from build123d import *

# Parameters (mm, degrees)
F0_W     = 41
F0_H     = 41
F1_DEPTH = 47
F2_R     = 1.25
F3_DEPTH = 25
F4_R     = 11
F5_DEPTH = 2
F6_R     = 2.25
F7_DEPTH = 21
F8_R     = 8
F9_DEPTH = 7


with BuildPart() as f1:
    # F0 (on Top) → F1 (new body)
    with BuildSketch(Plane.XY):
        with Locations((20.5, 20.5)):
            Rectangle(F0_W, F0_H)
    extrude(amount=F1_DEPTH)

    # F2 (on face) → F3 (cut)
    with BuildSketch(Plane.XY.offset(47)):
        with Locations((5, 5)):
            Circle(F2_R)
        with Locations((36, 5)):
            Circle(F2_R)
        with Locations((36, 36)):
            Circle(F2_R)
        with Locations((5, 36)):
            Circle(F2_R)
    extrude(amount=-F3_DEPTH, mode=Mode.SUBTRACT)

    # F4 (on face) → F5 (join)
    with BuildSketch(Plane.XY.offset(47)):
        with Locations((20.5, 20.5)):
            Circle(F4_R)
    extrude(amount=F5_DEPTH)

    # F6 (on face) → F7 (join)
    with BuildSketch(Plane.XY.offset(49)):
        with Locations((20.5, 20.5)):
            Circle(F6_R)
    extrude(amount=F7_DEPTH)

    # F8 (on face) → F9 (join)
    with BuildSketch(Plane.XY.offset(70)):
        with Locations((20.5, 20.5)):
            Circle(F8_R)
    extrude(amount=-F9_DEPTH)


solid = f1.part
Source: CAD feature listing. Evaluate the final solid. Frame: model axes, mm. A direction names the side the tool comes from. Give positions to 0.01 mm unless a question says otherwise; leave off trailing zeros. Order: outer loops, then holes, each group sorted by start corner. A loop starts at its lowest first (then second) coordinate and runs counter-clockwise, first axis right, second up. Notation, with made-up numbers: (-13, -10) -> (41, -10) arc R11 ccw to (41, 2) -> close; hole circle Ø8 at (-2, -33). An arc over 180 degrees is marked (long way). Use a Markdown table: item, result.
1) Section query A-A, the plane y = 5. Return the cut outline in (x, z).
Answer list:
| item | result |
|---|---|
| outline | (0, 0) -> (41, 0) -> (41, 47) -> (37.25, 47) -> (37.25, 22) -> (34.75, 22) -> (34.75, 47) -> (6.25, 47) -> (6.25, 22) -> (3.75, 22) -> (3.75, 47) -> (0, 47) -> close |
2) Reachability of faces 1 (the flat face through (0, 20, 23)), 2 (the flat face through (22.2, 18.8, 63)), 3 (the cylindrical face through (30.661, 16.287, 47.986)) from +Z, -Z, +X, -X, +Y, -Y: full face, straight path, thin tool, end or side. Return the list, or none.
Answer list:
| item | result |
|---|---|
| face 1 | +Z, -Z, -X, +Y, -Y |
| face 2 | none |
| face 3 | +Z |
3) Section query C-C, the plane x = 20.5. Return the cut outline in (y, z).
Answer list:
| item | result |
|---|---|
| outline | (0, 0) -> (41, 0) -> (41, 47) -> (31.5, 47) -> (31.5, 49) -> (22.75, 49) -> (22.75, 63) -> (28.5, 63) -> (28.5, 70) -> (12.5, 70) -> (12.5, 63) -> (18.25, 63) -> (18.25, 49) -> (9.5, 49) -> (9.5, 47) -> (0, 47) -> close |
4) Ray query, line 1 along Y through (x, z) = (5, 39); line 2 along Z through (x, y) = (15, 25); line 3 along Y through (x, z) = (4.5, 40). Return the intervals inside material, ascending. Write a range as [from, to].
Answer list:
| item | result |
|---|---|
| line 1 | [0, 3.75], [6.25, 34.75], [37.25, 41] |
| line 2 | [0, 49], [63, 70] |
| line 3 | [0, 3.85], [6.15, 34.85], [37.15, 41] |
5) Contact query for flat-ended pins moving along their axis: P1, Ø3, axis at x = 5, y = 36, coming from the +Z side; P2, Ø8, axis at x = 30, z = 7, coming from the -Y side; P3, Ø1.2, axis at x = 36, y = 5, coming from the +Z side; P4, Ø12, axis at y = 5.5, z = 62.5, coming from the -X side. Output: stop coordinate, or through.
Answer list:
| item | result |
|---|---|
| P1 | z = 47 |
| P2 | y = 0 |
| P3 | z = 22 |
| P4 | through |
6) Mould query, pull axis Y, two halves, no side actions, for faces 4 (the flat face through (20, 41, 23)), 5 (the cylindrical face through (21.538, 18.504, 55.902)), 6 (the cylindrical face through (4.73, 3.78, 34.67)). Classes: +Y half, -Y half, draft (parallel to the pull), parting line (faces both ways), or undercut.
Answer list:
| item | result |
|---|---|
| face 4 | +Y half |
| face 5 | parting line |
| face 6 | undercut |
7) Section query B-B, the plane x = 14. Return the cut outline in (y, z), then the cut area to 3 significant figures.
Answer list:
| item | result |
|---|---|
| outline | (0, 0) -> (41, 0) -> (41, 47) -> (29.37, 47) -> (29.37, 49) -> (11.63, 49) -> (11.63, 47) -> (0, 47) -> close; (15.84, 63) -> (25.16, 63) -> (25.16, 70) -> (15.84, 70) -> close |
| area | 2,030 mm² |
8) Section query D-D, the plane z = 62. Return the cut outline in (x, y), then the cut area to 3 significant figures.
Answer list:
| item | result |
|---|---|
| outline | circle Ø4.5 at (20.5, 20.5) |
| area | 15.9 mm² |
